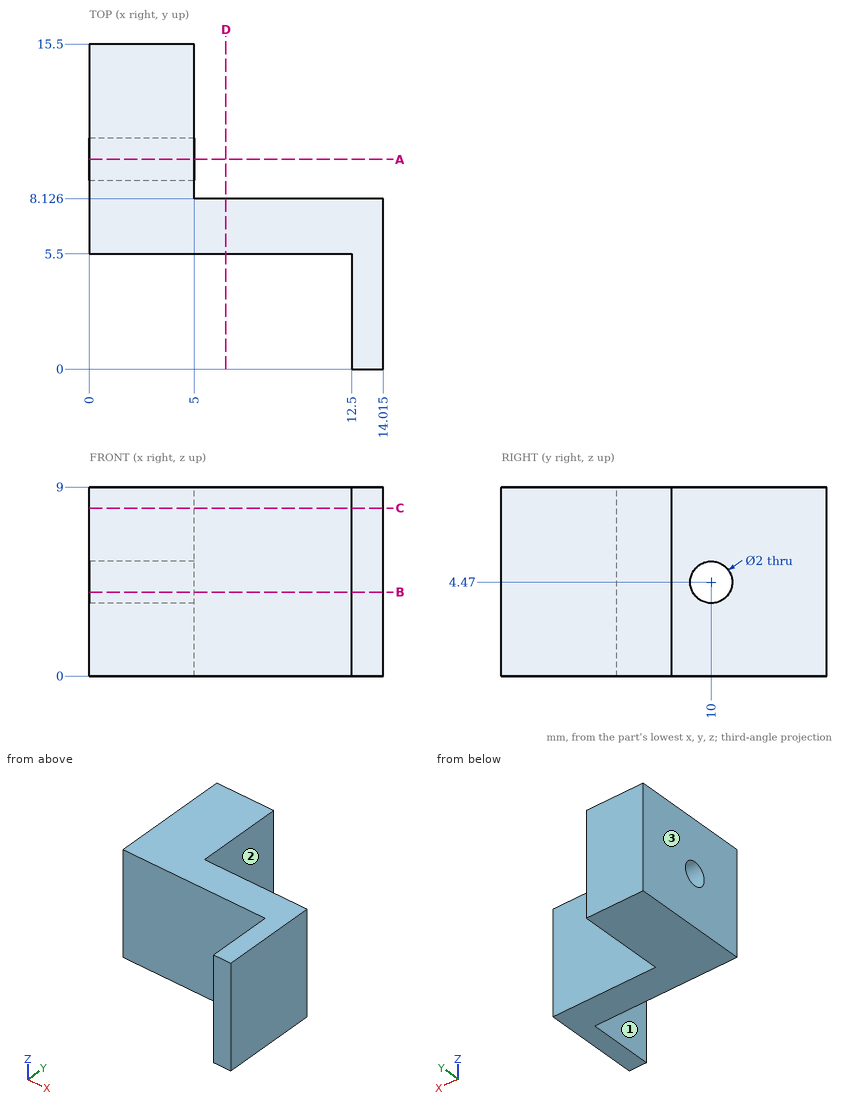
Source: three-view drawing plus pictorial views. Frame: mm from the lowest corner of the part. A direction names the side the tool comes from. Round coordinates to 2 decimals unless told otherwise and drop trailing zeros. Loops run counter-clockwise (first coordinate to the right, second up) from the corner with the lowest first, then second, coordinate; pieces in that order, holes last. Notation, with made-up numbers: (45.5, 37.5) - (95.5, 37.5) arc R30 cw to (95.5, 62.5) - close; hole circle Ø8 at (-11.75, 73.25). An arc over 180 degrees is marked (long way). Write each question's results on one line, items separated by ' | '. Start each with the question number.
1) Cut plane C-C on z = 8. Return loops of the section in (x, y) (1 decimal).
2) Cut plane B-B on z = 4. Return loops of the section in (x, y) (1 decimal).
3) Cut plane D-D on x = 6.5. Return loops of the section in (y, z), then the cut area to 3 significant figures.
4) First-contact query: P1, Ø2, axis at y = 10.5, z = 4, coming from the +X side; P2, Ø1.6, axis at y = 10, z = 4.47, coming from the -X side; P3, Ø5, axis at x = 6, y = 9, coming from the -Z side; P4, Ø1.5, axis at x = 4, z = 5, coming from the -Y side. Flat tips, straight axial feed; report the tip coordinate or a pass-through.
5) Line query: probe 1 along Z at (x, y) = (1.9, 10); probe 2 along X at (y, z) = (14.25, 7); probe 3 along Y at (x, z) = (10, 8.25). Output: solid intervals per line, ascending. Write a range as [from, to].
6) Access query for the marked faces 1, 2 and 3. Directions: +Z, -Z, +X, -X, +Y, -Y. A direction counts if a zero-diameter tool reaches every point of the face in a straight line with its end or side. Return the directions, or none.
7) Cut plane A-A on y = 10. Return loops of the section in (x, z), then the cut area to 3 significant figures.
Verdict:
1) outline: (0, 5.5) - (12.5, 5.5) - (12.5, 0) - (14, 0) - (14, 8.1) - (5, 8.1) - (5, 15.5) - (0, 15.5) - close
2) outline: (0, 5.5) - (12.5, 5.5) - (12.5, 0) - (14, 0) - (14, 8.1) - (5, 8.1) - (5, 9.1) - (0, 9.1) - close; (0, 10.9) - (5, 10.9) - (5, 15.5) - (0, 15.5) - close
3) outline: (5.5, 0) - (8.13, 0) - (8.13, 9) - (5.5, 9) - close | area: 23.6 mm2
4) P1: stops at x = 5 | P2: passes through | P3: stops at z = 0 | P4: stops at y = 5.5
5) probe 1: z = [0, 3.47], [5.47, 9] | probe 2: x = [0, 5] | probe 3: y = [5.5, 8.13]
6) face 1: +Z, -Z, -X, -Y | face 2: +Z, -Z, +X, +Y | face 3: +Z, -Z, -X, +Y, -Y
7) outline: (0, 0) - (5, 0) - (5, 3.47) - (0, 3.47) - close; (0, 5.47) - (5, 5.47) - (5, 9) - (0, 9) - close | area: 35.0 mm2
